Design review of the part built by this model. Coordinates are the model's own, in mm. Coordinates: 2 decimals unless noted, no trailing zeros. Write each loop counter-clockwise with the first axis right and the second up, starting at its lowest first coordinate (ties: lowest second). Pieces come first, ordered by that corner, then holes.
Q1. To check wall thickness, follow probe 1 along Y at (x, z) = (176, 0.9); probe 2 along X at (y, z) = (175, 0.7); probe 3 along Y at (x, z) = (75.5, 0.35). State the ranges of each line that lie inside material, in increasing order.
Q2. Add section B-B, the plane x = 85.5. Give the boundary of the cut face in (y, z), plus the area to 3 significant figures.
Q3. Add section A-A, the plane z = 1.3. Give the boundary of the cut face in (x, y), plus the area to 3 significant figures.
Q4. Clearance check with a flat-ended pin moving along its axis: pin 1 Ø0.6 at (x, z) = (91, 0.5) entering from +Y. State where the tip first meets the part, or that it passes through.
from build123d import *

# Parameters (mm, degrees)
SKETCH_1_W          = 184
SKETCH_1_H          = 182
EXTRUDE_1_DEPTH     = 2
M3X0_5_1_D          = 2.5
SKETCH_4_W          = 64
SKETCH_4_H          = 20
CUT_EXTRUDE_1_DEPTH = 259.812673569
SKETCH_6_W          = 64
SKETCH_6_H          = 22
CUT_EXTRUDE_2_DEPTH = 10


with BuildPart() as part:
    # ｽｹｯﾁ1 → ﾎﾞｽ - 押し出し1 (new body)
    with BuildSketch(Plane.XY):
        with Locations((92, 91)):
            Rectangle(SKETCH_1_W, SKETCH_1_H)
    extrude(amount=EXTRUDE_1_DEPTH)

    # M3x0.5 ねじ穴1 (through all)
    with Locations(Plane.XY.offset(2)):
        with Locations((8, 175), (8, 7), (176, 7), (176, 175)):
            Hole(M3X0_5_1_D / 2)

    # ｽｹｯﾁ4 → ｶｯﾄ - 押し出し1 (cut, through all)
    with BuildSketch(Plane(origin=(0, 0, 0), x_dir=(-1, 0, 0), z_dir=(0, 0, -1))):
        with Locations((-92, 172)):
            Rectangle(SKETCH_4_W, SKETCH_4_H)
    extrude(amount=-CUT_EXTRUDE_1_DEPTH, mode=Mode.SUBTRACT)

    # ｽｹｯﾁ6 → ｶｯﾄ - 押し出し2 (cut)
    with BuildSketch(Plane(origin=(0, 0, 0), x_dir=(-1, 0, 0), z_dir=(0, 0, -1))):
        with Locations((-92, 91)):
            Rectangle(SKETCH_6_W, SKETCH_6_H)
    extrude(amount=-CUT_EXTRUDE_2_DEPTH, mode=Mode.SUBTRACT)


solid = part.part
Here are the results:
1. probe 1: y = 0 to 5.75, 8.25 to 173.75, 176.25 to 182
1. probe 2: x = 0 to 6.75, 9.25 to 60, 124 to 174.75, 177.25 to 184
1. probe 3: y = 0 to 80, 102 to 162
2. outline: (0, 0) - (80, 0) - (80, 2) - (0, 2) - close; (102, 0) - (162, 0) - (162, 2) - (102, 2) - close
2. area: 280 mm2
3. outline: (0, 0) - (184, 0) - (184, 182) - (124, 182) - (124, 162) - (60, 162) - (60, 182) - (0, 182) - close; hole circle Ø2.5 at (8, 7); hole circle Ø2.5 at (8, 175); hole (60, 80) - (124, 80) - (124, 102) - (60, 102) - close; hole circle Ø2.5 at (176, 7); hole circle Ø2.5 at (176, 175)
3. area: 30,800 mm2
4. pin 1: stops at y = 162
